from build123d import *

# Parameters (mm, degrees)
F0_W     = 5.0798452705
F0_H     = 5.1181645604
F0_W_2   = 5.08
F0_H_2   = 5.08
F0_W_3   = 5.8267449073
F0_H_3   = 5.1171841682
F0_W_4   = 33.3881005645
F0_H_4   = 110.1423501968
F0_W_5   = 30.5098136887
F0_H_5   = 60.6358556543
F0_W_6   = 33.9637510478
F0_H_6   = 61.2115135882
F0_W_7   = 45.72
F0_W_8   = 14.9670690298
F0_H_7   = 47.5115125301
F1_DEPTH = 2.54
F2_DEPTH = 5.08
F5_D     = 1.27


# Not quite as in the source:
# - a feature of the source that left no trace in its solid (it failed there, or was rolled back) is left out
# - a feature names something its author has since deleted; it is built from what else it names


with BuildPart() as f1:
    # F0 (on Top) → F1 (new body)
    with BuildSketch(Plane.XY):
        Polygon((101.6, -60.96), (101.6, 60.96), (-8.89, 60.96), (-8.89, 55.88), (-13.97, 55.88), (-13.97, 60.96), (-83.82, 60.96), (-83.82, 55.88), (-88.9, 55.88), (-88.9, 60.96), (-101.6, 60.96), (-101.6, -60.96), align=None)
        Polygon((-91.44, -50.7502545385), (-85.6132550927, -50.7809177198), (-85.6132550927, -55.9297454615), (-91.44, -55.8990822802), align=None, mode=Mode.SUBTRACT)
        with Locations((-37.7266275464, -53.34)):
            Rectangle(F0_W, F0_H, mode=Mode.SUBTRACT)
        with Locations((-25.0266275464, -53.34)):
            Rectangle(F0_W_2, F0_H_2, mode=Mode.SUBTRACT)
        with Locations((-88.5266275464, -2.54)):
            Rectangle(F0_W_3, F0_H_3, mode=Mode.SUBTRACT)
        with Locations((-62.787938863, -1.0339058936)):
            Rectangle(F0_W_4, F0_H_4, mode=Mode.SUBTRACT)
        with Locations((-37.7266275464, -2.54)):
            Rectangle(F0_W_2, F0_H_2, mode=Mode.SUBTRACT)
        with Locations((-25.0266275464, -2.54)):
            Rectangle(F0_W_2, F0_H_2, mode=Mode.SUBTRACT)
        with Locations((25.7733724536, -53.34)):
            Rectangle(F0_W_2, F0_H_2, mode=Mode.SUBTRACT)
        with Locations((38.4733724536, -53.34)):
            Rectangle(F0_W_2, F0_H_2, mode=Mode.SUBTRACT)
        with Locations((89.2733724536, -53.34)):
            Rectangle(F0_W_2, F0_H_2, mode=Mode.SUBTRACT)
        with Locations((0.8221440949, -27.5141232414)):
            Rectangle(F0_W_5, F0_H_5, mode=Mode.SUBTRACT)
        with Locations((25.7733724536, -2.54)):
            Rectangle(F0_W_2, F0_H_2, mode=Mode.SUBTRACT)
        with Locations((38.4733724536, -2.54)):
            Rectangle(F0_W_2, F0_H_2, mode=Mode.SUBTRACT)
        with Locations((63.7606251985, -27.8019522084)):
            Rectangle(F0_W_6, F0_H_6, mode=Mode.SUBTRACT)
        with Locations((89.2733724536, -2.54)):
            Rectangle(F0_W_2, F0_H_2, mode=Mode.SUBTRACT)
        with Locations((-87.63, 10.16)):
            Rectangle(F0_W_2, F0_H_2, mode=Mode.SUBTRACT)
        with Locations((-5.08, 10.16)):
            Rectangle(F0_W_2, F0_H_2, mode=Mode.SUBTRACT)
        with Locations((-35.56, 15.24)):
            Rectangle(F0_W_2, F0_H_2, mode=Mode.SUBTRACT)
        with Locations((-35.56, 43.18)):
            Rectangle(F0_W_2, F0_H_2, mode=Mode.SUBTRACT)
        Polygon((-3.4952829592, 50.3914393485), (-3.4952829592, 55.88), (21.6417368501, 55.88), (21.6417368501, 15.0844864547), (-3.4952829592, 15.0844864547), (-3.4952829592, 21.6086003929), (-26.5215560794, 21.6086003929), (-26.5215560794, 50.3914393485), align=None, mode=Mode.SUBTRACT)
        with Locations((51.0222736127, 15.0563112164)):
            Rectangle(F0_W_7, F0_H_2, mode=Mode.SUBTRACT)
        with Locations((32.4802736127, 32.8363112164)):
            Rectangle(F0_W_2, F0_H_2, mode=Mode.SUBTRACT)
        with Locations((69.5642736127, 32.8363112164)):
            Rectangle(F0_W_2, F0_H_2, mode=Mode.SUBTRACT)
        with Locations((87.6503884792, 32.1242437349)):
            Rectangle(F0_W_8, F0_H_7, mode=Mode.SUBTRACT)
        with Locations((51.5818764424, 50.6163112164)):
            Rectangle(F0_W_7, F0_H_2, mode=Mode.SUBTRACT)
    extrude(amount=F1_DEPTH)

    # F0 (on Top) → F2 (join)
    with BuildSketch(Plane.XY):
        with Locations((-86.36, 58.42)):
            Rectangle(F0_W_2, F0_H_2)
        with Locations((-35.56, 43.18)):
            Rectangle(F0_W_2, F0_H_2)
        with Locations((-11.43, 58.42)):
            Rectangle(F0_W_2, F0_H_2)
        with Locations((-35.56, 15.24)):
            Rectangle(F0_W_2, F0_H_2)
        with Locations((-5.08, 10.16)):
            Rectangle(F0_W_2, F0_H_2)
        with Locations((-87.63, 10.16)):
            Rectangle(F0_W_2, F0_H_2)
        with Locations((-88.5266275464, -2.54)):
            Rectangle(F0_W_3, F0_H_3)
        with Locations((-37.7266275464, -2.54)):
            Rectangle(F0_W_2, F0_H_2)
        with Locations((-37.7266275464, -53.34)):
            Rectangle(F0_W, F0_H)
        with Locations((-25.0266275464, -2.54)):
            Rectangle(F0_W_2, F0_H_2)
        with Locations((25.7733724536, -2.54)):
            Rectangle(F0_W_2, F0_H_2)
        with Locations((38.4733724536, -2.54)):
            Rectangle(F0_W_2, F0_H_2)
        with Locations((89.2733724536, -2.54)):
            Rectangle(F0_W_2, F0_H_2)
        with Locations((89.2733724536, -53.34)):
            Rectangle(F0_W_2, F0_H_2)
        with Locations((38.4733724536, -53.34)):
            Rectangle(F0_W_2, F0_H_2)
        with Locations((25.7733724536, -53.34)):
            Rectangle(F0_W_2, F0_H_2)
        with Locations((-25.0266275464, -53.34)):
            Rectangle(F0_W_2, F0_H_2)
        Polygon((-85.6132550927, -55.9297454615), (-85.6132550927, -50.7809177198), (-91.44, -50.7502545385), (-91.44, -55.8990822802), align=None)
        with Locations((32.4802736127, 32.8363112164)):
            Rectangle(F0_W_2, F0_H_2)
        with Locations((51.0222736127, 15.0563112164)):
            Rectangle(F0_W_7, F0_H_2)
        with Locations((69.5642736127, 32.8363112164)):
            Rectangle(F0_W_2, F0_H_2)
        with Locations((51.5818764424, 50.6163112164)):
            Rectangle(F0_W_7, F0_H_2)
    extrude(amount=F2_DEPTH)

    # F5 (through all)
    with Locations(Plane(origin=(0, 0, 0), x_dir=(1, 0, 0), z_dir=(0, 0, -1))):
        with Locations((-25.0266275464, 2.54), (-37.7266275464, 2.54), (25.7733724536, 2.54), (38.4733724536, 2.54), (89.2733724536, 2.54), (89.2733724536, 53.34), (38.4733724536, 53.34), (25.7733724536, 53.34), (-25.0266275464, 53.34), (-37.7266275464, 53.34), (-88.5266275464, 53.34), (-88.5266275464, 2.54), (-87.63, -10.16), (-35.56, -15.24), (-5.08, -10.16), (32.4802736127, -32.8363112164), (69.5642736127, -32.8363112164), (-11.43, -58.42), (-35.56, -43.18), (-86.36, -58.42)):
            Hole(F5_D / 2)


solid = f1.part
Could you check a few things on this model? Use its own coordinates, in mm. Coordinates: 2 decimals unless noted, no trailing zeros. Write each loop counter-clockwise with the first axis right and the second up, starting at its lowest first coordinate (ties: lowest second). Pieces come first, ordered by that corner, then holes. Notation, with made-up numbers: (9, 51.5) - (44, 51.5) arc R15 ccw to (44, 61.5) - close; hole circle Ø2 at (37.25, 33). An arc over 180 degrees is marked (long way). Put each result on its own line as item: value. Start each with the question number.
Q1. I want a section at B-B on x = -76.5. Write out the boundary of the cut face in (y, z), plus the area to 3 significant figures.
Q2. I'm going to push flat-ended pins straight in: P1, Ø1.3, axis at x = 89.5, z = 3.5, coming from the +Y side; P2, Ø3, axis at x = 74, z = 4.5, coming from the -Y side; P3, Ø3, axis at x = -14.5, y = 19, coming from the +Z side; P4, Ø1, axis at x = -11.43, y = 58.42, coming from the -Z side. Where does each tip first touch, or does it pass through?
Q3. Please list where these lines run through material, in increasing order: L1, parallel to X at y = 22.5, z = 1.1; L2, parallel to X at y = -16, z = 0.25; L3, parallel to X at y = 15.24, z = 1.7 (3 decimals).
Q4. Thinking about a two-plate mould opening in Y: for faces 1 (the flat face through (33, 32, 5.08)), 2 (the flat face through (-1, 60.96, 1)), 3 (the flat face through (-1, 14, 2.54)), which applies, pulls with the +Y half, pulls with the -Y half, needs draft (parallel to the pull), parting line crosses it, or undercut?
Q5. I want a section at C-C on z = 4.3. Count the separate pieces of the cut face and the enclosed holes in it, plus the area to 3 significant figures.
Q6. I want a section at A-A on y = -45. Write out the boundary of the cut face in (x, z), plus the area to 3 significant figures.
Checks:
1. outline: (-60.96, 0) - (-56.11, 0) - (-56.11, 2.54) - (-60.96, 2.54) - close; (54.04, 0) - (60.96, 0) - (60.96, 2.54) - (54.04, 2.54) - close
1. area: 29.9 mm²
2. P1: y = 0
2. P2: y = 12.52
2. P3: z = 2.54
2. P4: through
3. L1: -101.6 to -79.48, -46.09 to -26.52, 21.64 to 80.17, 95.13 to 101.6
3. L2: -101.6 to -79.48, -46.09 to -14.43, 16.08 to 46.78, 80.74 to 101.6
3. L3: -101.6 to -79.482, -46.094 to -36.195, -34.925 to -3.495, 21.642 to 80.167, 95.134 to 101.6
4. face 1: needs draft
4. face 2: pulls with the +Y half
4. face 3: undercut
5. separate pieces: 22
5. enclosed holes: 20
5. area: 964 mm²
6. outline: (-101.6, 0) - (-79.48, 0) - (-79.48, 2.54) - (-101.6, 2.54) - close; (-46.09, 0) - (-14.43, 0) - (-14.43, 2.54) - (-46.09, 2.54) - close; (16.08, 0) - (46.78, 0) - (46.78, 2.54) - (16.08, 2.54) - close; (80.74, 0) - (101.6, 0) - (101.6, 2.54) - (80.74, 2.54) - close
6. area: 268 mm²
